Autodesk Fusion 360 part; units mm, degrees
sketch "main body" plane through (0, 0, 0) normal (0, 0, 1) x (1, 0, 0)
  line L0 (7.7, -8.35) -> (-7.7, -8.35)
  line L1 (-7.7, -8.35) -> (-7.7, 8.35)
  line L2 (-7.7, 8.35) -> (7.7, 8.35)
  line L3 (7.7, 8.35) -> (7.7, -8.35)
  line L4 (7.7, -8.35) -> (-7.7, 8.35) construction
  line L5 (-7.7, -8.35) -> (7.7, 8.35) construction
  dimension "d1" = 15.4
  dimension "d2" = 16.7
extrude "Extrude1" add sketch "main body" along normal blind 6.6
sketch "top actuator" plane through (0, 0, 6.6) normal (0, 0, 1) x (-1, 0, 0)
  line L0 (-7.7, -8.35) -> (7.7, -8.35)
  line L1 (7.7, -8.35) -> (7.7, 8.35)
  line L2 (7.7, 8.35) -> (-7.7, 8.35)
  line L3 (-7.7, 8.35) -> (-7.7, -8.35)
  circle A0 centre (0, -2.35) radius 2.725
  dimension "d5" = 5.45
  dimension "d6" = 6
extrude "Extrude2" add sketch "top actuator" along normal blind 2 contours A0
fillet "Fillet1" radius 0.5 4 edges at (-7.7, -8.35, 3.3) (7.7, 8.35, 3.3) (7.7, -8.35, 3.3) (-7.7, 8.35, 3.3)
sketch "side cuts" plane through (-7.7, 0, 0) normal (-1, 0, 0) x (0, -1, 0)
  line L0 (-7.85, 6.6) -> (-7.85, 0)
  line L1 (-7.85, 0) -> (7.85, 0)
  line L2 (7.85, 0) -> (7.85, 6.6)
  line L3 (7.85, 6.6) -> (-7.85, 6.6)
  line L4 (-8.35, 0) -> (-8.35, 6.6)
  line L5 (-8.35, 6.6) -> (-8.35, 0)
  line L6 (0.375, 8.6) -> (-5.075, 8.6)
  line L7 (-2.35, 8.6) -> (-2.35, 0) construction
  line L8 (-1.1, 4.1) -> (-3.6, 4.1)
  line L9 (-3.6, 4.1) -> (-3.6, 6.6)
  line L10 (-3.6, 6.6) -> (-1.1, 6.6)
  line L11 (-1.1, 6.6) -> (-1.1, 4.1)
  line L12 (-1.1, 4.1) -> (-3.6, 6.6) construction
  line L13 (-3.6, 4.1) -> (-1.1, 6.6) construction
  line L14 (-1.1, 0) -> (-3.6, 0)
  line L15 (-3.6, 0) -> (-3.6, 1.8)
  line L16 (-3.6, 1.8) -> (-1.1, 1.8)
  line L17 (-1.1, 1.8) -> (-1.1, 0)
  line L18 (-1.1, 0) -> (-3.6, 1.8) construction
  line L19 (-3.6, 0) -> (-1.1, 1.8) construction
  point P0 (-2.35, 5.35)
  point P1 (-2.35, 0.9)
  dimension "d10" = 8.6
  dimension "d11" = 2.5
  dimension "d12" = 2.5
  dimension "d13" = 2.5
  dimension "d14" = 1.8
extrude "Extrude3" cut sketch "side cuts" against normal blind 0.6 contours L3 L8 L9 L10 L11 | L1 L14 L15 L16 L17
mirror "Mirror1" about plane through (0, 0, 0) normal (1, 0, 0) of "Extrude3"
sketch "Sketch4" plane through (0, -8.35, 0) normal (0, -1, 0) x (1, 0, 0)
  line L0 (7.2, 0) -> (7.2, 6.6)
  line L1 (7.2, 6.6) -> (-7.2, 6.6)
  line L2 (-7.2, 6.6) -> (-7.2, 0)
  line L3 (-7.2, 0) -> (7.2, 0)
  line L4 (-7.2, 2.9) -> (7.2, 2.9) construction
  circle A0 centre (-5, 4.6) radius 2
  line L5 (0, 6.6) -> (0, 0) construction
  line L6 (-7, 4.6) -> (-3, 4.6)
  line L7 (-3, 4.6) -> (-3, 1.7)
  line L8 (-3, 1.7) -> (-7, 1.7)
  line L9 (-7, 1.7) -> (-7, 4.6)
  line L10 (-3, 1.7) -> (0, 1.7)
  line L11 (0, 1.7) -> (0, 4.15)
  line L12 (0, 4.15) -> (-3, 4.15)
  line L13 (-3, 4.15) -> (-3, 1.7)
  circle A1 centre (-5, 4.6) radius 1
  circle A2 centre (0, 1.5) radius 1
  circle A3 centre (0, 1.5) radius 1.5
  circle A4 centre (5, 4.6) radius 2
  circle A5 centre (5, 4.6) radius 1
  line L14 (7, 1.7) -> (7, 4.6)
  line L15 (3, 1.7) -> (7, 1.7)
  line L16 (3, 4.6) -> (3, 1.7)
  line L17 (0, 4.15) -> (3, 4.15)
  line L18 (3, 1.7) -> (0, 1.7)
  dimension "d18" = 3.7
  dimension "d19" = 4
  dimension "d20" = 5
  dimension "d21" = 1.7
  dimension "d22" = 2
  dimension "d23" = 2.45
  dimension "d24" = 3
  dimension "d25" = 2
  dimension "d26" = 2
  dimension "d27" = 3
extrude "Extrude4" add sketch "Sketch4" along normal blind 1.5 contours L10 A2 A3 L18 | A4 | L10 L11 A2 A3 | L7 L10 L11 L12 L13 A3 | A0 L6 A1 | A4 L14 L15 L16 | A0 L7 L8 L9 L13 | L11 A2 A3 L18 | L11 A3 L16 L17 L18 | A0 L6 A1
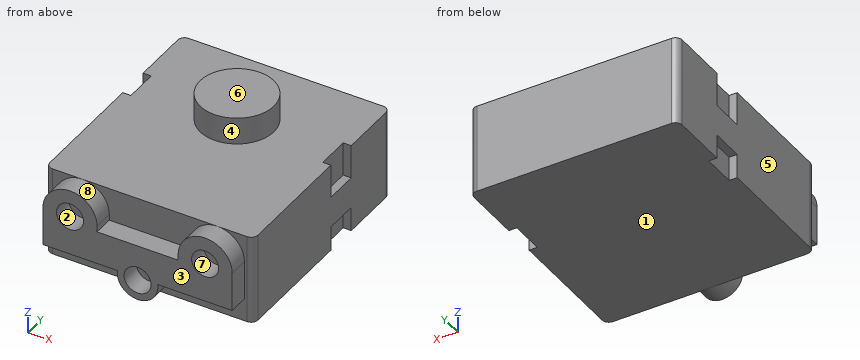
Source: CAD feature listing. Evaluate the final solid. Frame: model axes, mm. Face numbers are marked on the shaded views. A direction names the side the tool comes from. Round coordinates to 2 decimals unless told otherwise and drop trailing zeros. Order: outer loops, then holes, each group sorted by start corner. A loop starts at its lowest first (then second) coordinate and runs counter-clockwise, first axis right, second up. Notation, with made-up numbers: (-25, 37.5) - (2, 37.5) arc R30 ccw to (2, 76.5) - close; hole circle Ø6 at (-4.5, 74). An arc over 180 degrees is marked (long way). Use a Markdown table: item, result. Add a question column.
1. Set-up query: the marked faces 4, 5, 6, 7 and 8. Return all of +Z, -Z, +X, -X, +Y, -Y with unobstructed straight access to the full face (end or side cutting, diameter ignored); none if empty.
2. Mould query, pull axis Z, two halves, no side actions, for the marked faces 1, 2 and 3. Classes: +Z half, -Z half, draft (parallel to the pull), parting line (faces both ways), or undercut.
3. Section query B-B (z = 7). Return the cut outline in (x, y) (3 decimals), then the cut area to 3 significant figures.
4. Line query: probe 1 along Z at (x, y) = (0, -8.75); probe 2 along X at (y, z) = (-9.2, 1.5); probe 3 along Y at (x, z) = (-2, 5). Output: solid intervals per line, ascending.
5. Section query A-A (y = 2.35). Return the cut outline in (x, z) (3 decimals).
6. Section query C-C (x = -5.5). Return the cut outline in (y, z), then the cut area to 3 significant figures.
7. Section query D-D (y = -3.25). Return the cut outline in (x, z), then the cut area to 3 significant figures.
8. First-contact query: pin 1 (0.7 mm diameter, centred on x = 7.5, z = 1, fed in from -Y); pin 2 (0.5 mm diameter, centred on x = -7.5, y = 2, fed in from -Z); pin 3 (1.6 mm diameter, centred on y = -9.5, z = 3, fed in from +X). Flat tips, straight axial feed; report the tip coordinate or a pass-through.
Derived:
| question | item | result |
|---|---|---|
| 1 | face 4 | +Z |
| 1 | face 5 | +Z, -Z, -X, +Y, -Y |
| 1 | face 6 | +Z, +X, -X, +Y, -Y |
| 1 | face 7 | -Y |
| 1 | face 8 | +Z, -Y |
| 2 | face 1 | -Z half |
| 2 | face 2 | undercut |
| 2 | face 3 | draft |
| 3 | outline | circle Ø5.45 at (0, 2.35) |
| 3 | area | 23.3 mm2 |
| 4 | probe 1 | 0 to 0.5, 2.5 to 4.15 |
| 4 | probe 2 | -1.5 to -1, 1 to 1.5 |
| 4 | probe 3 | -8.35 to 8.35 |
| 5 | outline | (-7.7, 1.8) - (-7.1, 1.8) - (-7.1, 0) - (7.1, 0) - (7.1, 1.8) - (7.7, 1.8) - (7.7, 4.1) - (7.1, 4.1) - (7.1, 6.6) - (2.725, 6.6) - (2.725, 8.6) - (-2.725, 8.6) - (-2.725, 6.6) - (-7.1, 6.6) - (-7.1, 4.1) - (-7.7, 4.1) - close |
| 6 | outline | (-9.85, 1.7) - (-8.35, 1.7) - (-8.35, 0) - (8.35, 0) - (8.35, 6.6) - (-8.35, 6.6) - (-8.35, 6.54) - (-9.85, 6.54) - (-9.85, 5.47) - (-8.35, 5.47) - (-8.35, 3.73) - (-9.85, 3.73) - close |
| 6 | area | 115 mm2 |
| 7 | outline | (-7.7, 0) - (7.7, 0) - (7.7, 6.6) - (-7.7, 6.6) - close |
| 7 | area | 102 mm2 |
| 8 | pin 1 | y = -8.35 |
| 8 | pin 2 | z = 1.8 |
| 8 | pin 3 | x = 7 |
